Model file for the job. Use its own axes, mm. Give positions to 0.01 mm unless a question says otherwise; leave off trailing zeros. Loops run counter-clockwise (first coordinate to the right, second up) from the corner with the lowest first, then second, coordinate; pieces in that order, holes last. Notation, with made-up numbers: M -37,-7.5 L 18,-7.5 A26 cw 18,17.5 Z; hole C 34,42.25 d8. An arc over 180 degrees is marked long. Answer in a Markdown table with one row per item.
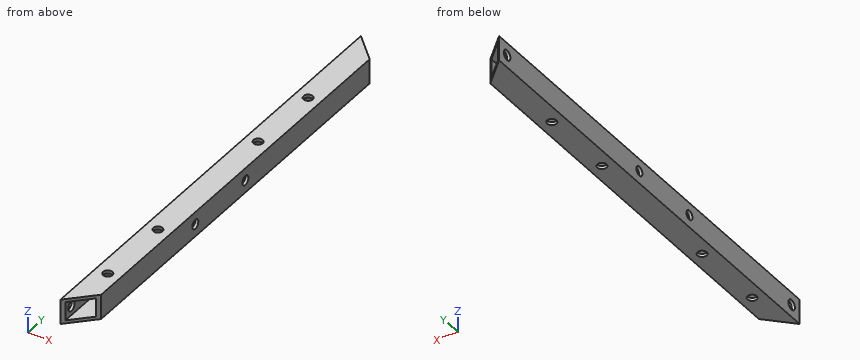
```python
from build123d import *

# Parameters (mm, degrees)
SKETCH_1_W          = 8
SKETCH_1_H          = 8
SKETCH_1_W_2        = 6
SKETCH_1_H_2        = 6
EXTRUDE_1_DEPTH     = 150
SKETCH_2_R          = 1.5
CUT_EXTRUDE_1_DEPTH = 10
CUT_EXTRUDE_2_DEPTH = 10
SKETCH_5_R          = 1.5
CUT_EXTRUDE_3_DEPTH = 10
SKETCH_6_R          = 1.625
CUT_EXTRUDE_4_DEPTH = 10


with BuildPart() as part:
    # 草图1 → 凸台-拉伸1 (new body)
    with BuildSketch(Plane(origin=(0, 0, 0), x_dir=(1, 0, 0), z_dir=(0, 1, 0))):
        Rectangle(SKETCH_1_W, SKETCH_1_H)
        Rectangle(SKETCH_1_W_2, SKETCH_1_H_2, mode=Mode.SUBTRACT)
    extrude(amount=EXTRUDE_1_DEPTH)

    # 草图2 → 切除-拉伸1 (cut)
    with BuildSketch(Plane(origin=(4, 0, 0), x_dir=(0, 0, -1), z_dir=(1, 0, 0))):
        with Locations((0, 80)):
            Circle(SKETCH_2_R)
        with Locations((0, 55)):
            Circle(SKETCH_2_R)
    extrude(amount=-CUT_EXTRUDE_1_DEPTH, mode=Mode.SUBTRACT)

    # 草图3 → 切除-拉伸2 (cut)
    with BuildSketch(Plane(origin=(0, 0, -4), x_dir=(-1, 0, 0), z_dir=(0, 0, -1))):
        Polygon((4, 150), (-4, 142), (-4, 150), align=None)
        Polygon((4, 0), (-4, 8), (-4, 0), align=None)
    extrude(amount=-CUT_EXTRUDE_2_DEPTH, mode=Mode.SUBTRACT)

    # 草图5 → 切除-拉伸3 (cut)
    with BuildSketch(Plane.XY.offset(4)):
        with Locations((0, 42.5)):
            Circle(SKETCH_5_R)
        with Locations(Location((0, 92.5, 0), (0, 0, 180))):
            Circle(SKETCH_5_R)
        with Locations((0, 117.5)):
            Circle(SKETCH_5_R)
        with Locations((0, 17.5)):
            Circle(SKETCH_5_R)
    extrude(amount=-CUT_EXTRUDE_3_DEPTH, mode=Mode.SUBTRACT)

    # 草图6 → 切除-拉伸4 (cut)
    with BuildSketch(Plane(origin=(-3, 0, 0), x_dir=(0, 0, -1), z_dir=(1, 0, 0))):
        with Locations((0, 146)):
            Circle(SKETCH_6_R)
        with Locations((0, 4)):
            Circle(SKETCH_6_R)
    extrude(amount=-CUT_EXTRUDE_4_DEPTH, mode=Mode.SUBTRACT)


solid = part.part
```
Q1. Drop flat-ended pins along their axis: pin 1 (2 mm diameter, centred on x = -1, z = 0, fed in from +Y); pin 2 (1.5 mm diameter, centred on x = -3, z = -2.5, fed in from +Y); pin 3 (3 mm diameter, centred on x = 1, z = 3, fed in from +Y). Give the stop position or say it passes through.
Reported:
| item | result |
|---|---|
| pin 1 | through |
| pin 2 | y = 149.75 |
| pin 3 | y = 146.5 |
Q2. Saw through at C-C (y = 110). Give the cut face in (x, z), and give its area (3 significant figures).
Reported:
| item | result |
|---|---|
| outline | M -4,-4 L 4,-4 L 4,4 L -4,4 Z; hole M -3,-3 L 3,-3 L 3,3 L -3,3 Z |
| area | 28.0 mm² |
Q3. Saw through at A-A (y = 80). Give the cut face in (x, z), and give its area (3 significant figures).
Reported:
| item | result |
|---|---|
| outline | M -4,-4 L 4,-4 L 4,-1.5 L 3,-1.5 L 3,-3 L -3,-3 L -3,-1.5 L -4,-1.5 Z; M -4,1.5 L -3,1.5 L -3,3 L 3,3 L 3,1.5 L 4,1.5 L 4,4 L -4,4 Z |
| area | 22.0 mm² |
Q4. Probe probe 1 along Z at (x, y) = (1.5, 106); probe 2 along Z at (x, y) = (-3.25, 80). List the from-to ranges inside material, lowest first.
Reported:
| item | result |
|---|---|
| probe 1 | -4 to -3, 3 to 4 |
| probe 2 | -4 to -1.5, 1.5 to 4 |
Q5. Saw through at B-B (z = 0). Give the number of separate pieces and of enclosed holes in the cut face, and give its area (4 significant figures).
Reported:
| item | result |
|---|---|
| separate pieces | 8 |
| enclosed holes | 0 |
| area | 265.5 mm² |
